Check sheet for the drawn part. Datum: minimum x, y, z corner. Units: mm. A direction names the side the tool comes from. Coordinates: 2 decimals unless noted, no trailing zeros. Write each loop counter-clockwise with the first axis right and the second up, starting at its lowest first coordinate (ties: lowest second). Pieces come first, ordered by that corner, then holes. Notation, with made-up numbers: M 23.25,54 L 39.25,54 A26 ccw 39.25,89 Z; hole C 4,-29 d2. An arc over 180 degrees is marked long. Answer in a Markdown table with one row per item.
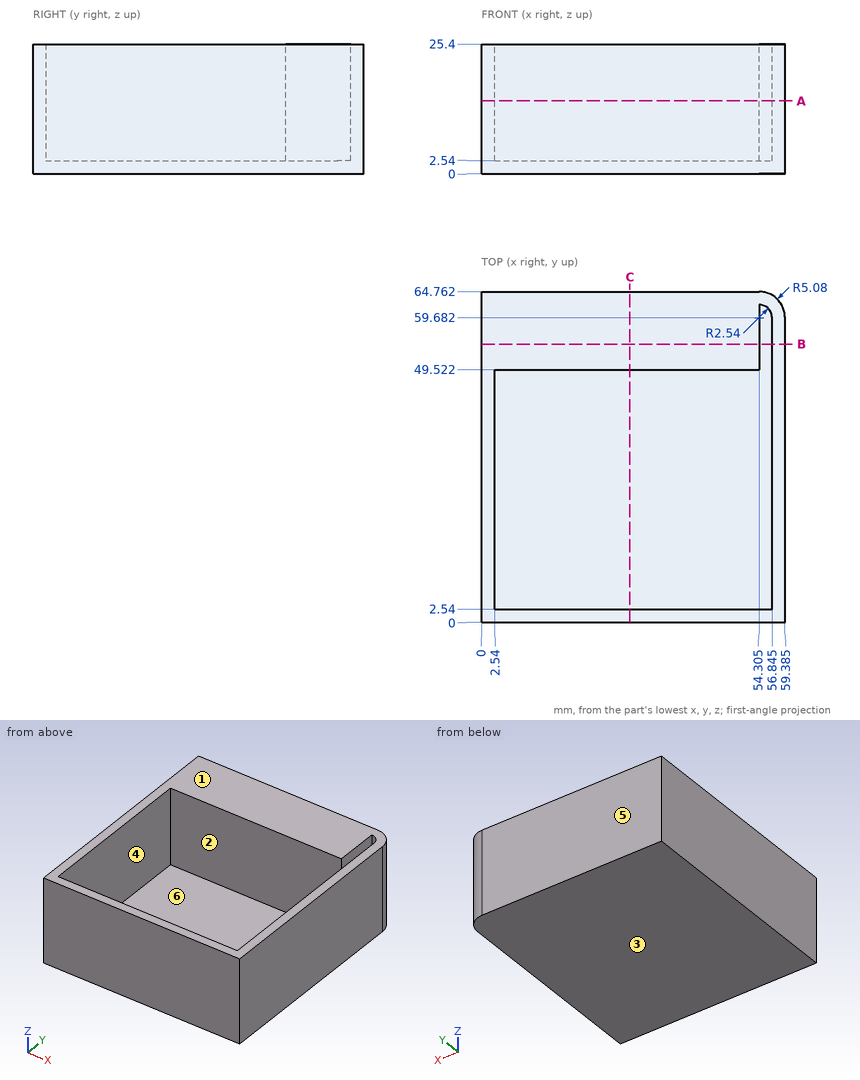
1) Tool access check on the marked faces 1 and 2. Record the directions out of +Z, -Z, +X, -X, +Y, -Y that give a thin tool (end or side, any length) a straight path to the whole face; none if there is none.
Response values:
| item | result |
|---|---|
| face 1 | +Z, +X, -X, +Y, -Y |
| face 2 | +Z |
2) Depth check by flat-ended pin: pin 1 (1 mm diameter, centred on x = 9.5, y = 21.5, fed in from +Z). Enter the tip coordinate at first touch or a pass-through.
Response values:
| item | result |
|---|---|
| pin 1 | stops at z = 2.54 |
3) Release check for a two-part mould opening along Y. For the marked faces 3, 4, 5 and 6 record: +Y half, -Y half, draft (parallel to the pull), parting line (faces both ways), or undercut.
Response values:
| item | result |
|---|---|
| face 3 | draft |
| face 4 | undercut |
| face 5 | +Y half |
| face 6 | undercut |
4) Sectioned sample at A-A (z = 14.25). Record the cut outline in (x, y) (1 decimal), then the cut area to 3 significant figures.
Response values:
| item | result |
|---|---|
| outline | M 0,0 L 59.4,0 L 59.4,59.7 A5.1 ccw 54.3,64.8 L 0,64.8 Z; hole M 2.5,2.5 L 56.8,2.5 L 56.8,59.7 A2.5 ccw 54.3,62.2 L 54.3,49.5 L 2.5,49.5 Z |
| area | 1,260 mm² |
5) Sectioned sample at C-C (x = 29). Record the cut outline in (y, z), then the cut area to 3 significant figures.
Response values:
| item | result |
|---|---|
| outline | M 0,0 L 64.76,0 L 64.76,25.4 L 49.52,25.4 L 49.52,2.54 L 2.54,2.54 L 2.54,25.4 L 0,25.4 Z |
| area | 571 mm² |
6) Thickness scan on L1, parallel to X at y = 41, z = 9 (1 decimal); L2, parallel to Y at x = 24.5, z = 18.25; L3, parallel to X at y = 55, z = 22 (1 decimal). Record the ranges inside material, lowest first. Write a range as [from, to].
Response values:
| item | result |
|---|---|
| L1 | x = [0, 2.5], [56.8, 59.4] |
| L2 | y = [0, 2.54], [49.52, 64.76] |
| L3 | x = [0, 54.3], [56.8, 59.4] |
7) Sectioned sample at B-B (y = 54.5). Record the cut outline in (x, z) (1 decimal), then the cut area to 3 significant figures.
Response values:
| item | result |
|---|---|
| outline | M 0,0 L 59.4,0 L 59.4,25.4 L 56.8,25.4 L 56.8,2.5 L 54.3,2.5 L 54.3,25.4 L 0,25.4 Z |
| area | 1,450 mm² |
